from build123d import *

# Parameters (mm, degrees)
SKETCH3_W          = 3
SKETCH3_H          = 1.001019848
CUT_EXTRUDE1_DEPTH = 50


with BuildPart() as part:
    # Sketch2 → Revolve1 (revolve)
    with BuildSketch(Plane.XY):
        Polygon((10.441459651, 6), (25.219960982, 6), (33.73435287, 6), (34.441459651, 5.292893219), (34.441459651, 2.788575112), (34.441459651, 0), (4.441459651, 0), (4.441459651, 12), align=None)
    revolve(axis=Axis((-22.000325263, 0, 0), (1, 0, 0)))

    # Sketch3 → Cut-Extrude1 (cut, symmetric)
    with BuildSketch(Plane(origin=(0, 0, 0), x_dir=(1, 0, 0), z_dir=(0, 1, 0))):
        with Locations((5.941459651, 0.500509924)):
            Rectangle(SKETCH3_W, SKETCH3_H)
    extrude(amount=CUT_EXTRUDE1_DEPTH, both=True, mode=Mode.SUBTRACT)


solid = part.part
Check sheet for the modelled part. Datum: model origin and axes. Units: mm. A direction names the side the tool comes from. Round coordinates to 2 decimals unless told otherwise and drop trailing zeros. Loops run counter-clockwise (first coordinate to the right, second up) from the corner with the lowest first, then second, coordinate; pieces in that order, holes last. Notation, with made-up numbers: M -1.5,77.25 L 17.5,77.25 A23 ccw 17.5,94.25 Z; hole C 0.25,38 d7. An arc over 180 degrees is marked long. One line per item, written item: value.
(1) Access from +Z, -Z, +X, -X, +Y, -Y to the whole of each face (thin tool, end or side, straight path). Record for faces 1 (the face through (6, 0, 0)), 2 (the face through (4.441, 0, 5)), 3 (the face through (22, -6, 0)).
Computed values:
face 1: -X, +Y, -Y
face 2: +Z, -Z, -X, +Y, -Y
face 3: +X
(2) Depth check by flat-ended pin: pin 1 Ø0.9 at (x, y) = (6, 2.5) entering from -Z; pin 2 Ø4 at (x, y) = (17, -3) entering from +Z; pin 3 Ø1.5 at (x, z) = (13.5, 5) entering from +Y. Enter the tip coordinate at first touch or a pass-through.
Computed values:
pin 1: stops at z = -10.61
pin 2: stops at z = 5.92
pin 3: stops at y = 4.24
(3) Sectioned sample at A-A, the plane y = 0. Record the cut outline in (x, z).
Computed values:
outline: M 4.44,-12 L 10.44,-6 L 33.73,-6 L 34.44,-5.29 L 34.44,5.29 L 33.73,6 L 10.44,6 L 4.44,12 L 4.44,0 L 7.44,0 L 7.44,-1 L 4.44,-1 Z
(4) Release check for a two-part mould opening along Z. For faces 4 (the face through (7.441, 0.1, -0.5)), 5 (the face through (34.441, 0, 0)), 6 (the face through (10.15, -1.36, -6.14)) record: +Z half, -Z half, draft (parallel to the pull), parting line (faces both ways), or undercut.
Computed values:
face 4: undercut
face 5: draft
face 6: parting line
(5) Sectioned sample at B-B, the plane x = 16. Record the cut outline in (y, z).
Computed values:
outline: C 0,0 d12
(6) Thickness scan on line 1 (Y direction, x = 18, z = -0.25); line 2 (X direction, y = 0.5, z = -0.75); line 3 (Y direction, x = 19, z = -3.5). Record the ranges inside material, lowest first.
Computed values:
line 1: y = -5.99 to 5.99
line 2: x = 7.44 to 34.44
line 3: y = -4.87 to 4.87
